```python
from build123d import *

# Parameters (mm, degrees)
SKETCH1_W           = 31.75
SKETCH1_H           = 8
SKETCH1_R           = 2.1
BOSS_EXTRUDE1_DEPTH = 21
SKETCH4_R           = 2.1
CUT_EXTRUDE3_DEPTH  = 38.5
SKETCH6_R           = 2.1
BOSS_EXTRUDE3_DEPTH = 2
SKETCH7_R           = 2.1
BOSS_EXTRUDE4_DEPTH = 2


with BuildPart() as part:
    # Sketch1 → Boss-Extrude1 (new body)
    with BuildSketch(Plane(origin=(0, 0, 0), x_dir=(1, 0, 0), z_dir=(0, 1, 0))):
        with Locations((4.725, 0)):
            Rectangle(SKETCH1_W, SKETCH1_H)
        with Locations(Location((0, 0, 0), (0, 0, 90))):
            Circle(SKETCH1_R, mode=Mode.SUBTRACT)
        with Locations(Location((-7.15, 0, 0), (0, 0, 90))):
            Circle(SKETCH1_R, mode=Mode.SUBTRACT)
        with Locations(Location((9.45, 0, 0), (0, 0, 90))):
            Circle(SKETCH1_R, mode=Mode.SUBTRACT)
        with Locations(Location((16.6, 0, 0), (0, 0, 90))):
            Circle(SKETCH1_R, mode=Mode.SUBTRACT)
    extrude(amount=BOSS_EXTRUDE1_DEPTH)

    # Sketch4 → Cut-Extrude3 (cut)
    with BuildSketch(Plane(origin=(20.6, 0, 0), x_dir=(0, 0, -1), z_dir=(1, 0, 0))):
        with Locations((0, 4)):
            Circle(SKETCH4_R)
    extrude(amount=-CUT_EXTRUDE3_DEPTH, mode=Mode.SUBTRACT)

    # Sketch6 → Boss-Extrude3 (add)
    with BuildSketch(Plane.XZ):
        with Locations(Location((-7.15, 0, 0), (0, 0, 90))):
            Circle(SKETCH6_R)
        with Locations(Location((0, 0, 0), (0, 0, 90))):
            Circle(SKETCH6_R)
        with Locations(Location((9.45, 0, 0), (0, 0, 90))):
            Circle(SKETCH6_R)
        with Locations(Location((16.6, 0, 0), (0, 0, 90))):
            Circle(SKETCH6_R)
    extrude(amount=-BOSS_EXTRUDE3_DEPTH)

    # Sketch7 → Boss-Extrude4 (add)
    with BuildSketch(Plane(origin=(20.6, 0, 0), x_dir=(0, 0, -1), z_dir=(1, 0, 0))):
        with Locations((0, 4)):
            Circle(SKETCH7_R)
    extrude(amount=-BOSS_EXTRUDE4_DEPTH)


solid = part.part
```
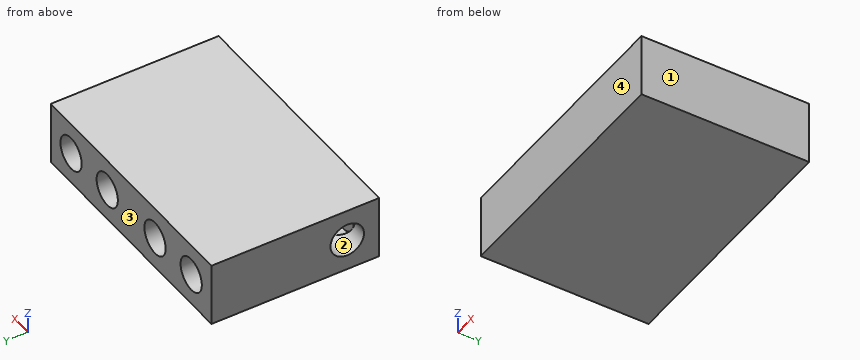
Input: part model. Units: mm. Frame: model coordinates. Face numbers are marked on the shaded views. Coordinates: 2 decimals unless noted, no trailing zeros. Write each loop counter-clockwise with the first axis right and the second up, starting at its lowest first coordinate (ties: lowest second). Pieces come first, ordered by that corner, then holes. Notation, with made-up numbers: (78, -2.75) -> (115, -2.75) arc R13 ccw to (115, 4.25) -> close; hole circle Ø4 at (-15.75, 78). An arc over 180 degrees is marked (long way). Answer as a JSON object with one key per item and string values.
1. Section A-A on y = 13.5. Return the cut outline in (x, z).
Result set:
{"outline": "(-11.15, -4) -> (20.6, -4) -> (20.6, 4) -> (-11.15, 4) -> close; hole circle Ø4.2 at (-7.15, 0); hole circle Ø4.2 at (0, 0); hole circle Ø4.2 at (9.45, 0); hole circle Ø4.2 at (16.6, 0)"}
2. Material intervals for line 1 (X direction, y = 11, z = 0); line 2 (Z direction, x = 15, y = 4); line 3 (X direction, y = 9.5, z = 0.5), sorted ascending. Write a range as from..to.
Result set:
{"line 1": "x = -11.15..-9.25, -5.05..-2.1, 2.1..7.35, 11.55..14.5, 18.7..20.6", "line 2": "z = -4..-2.1, 2.1..4", "line 3": "x = -11.15..-9.19, -5.11..-2.04, 2.04..7.41, 11.49..14.56, 18.64..20.6"}
3. Section D-D on z = 0. Count the separate pieces of the cut face and the enclosed holes in it, then the cut area to 3 significant figures.
Result set:
{"separate pieces": "5", "enclosed holes": "0", "area": "293 mm2"}
4. Section C-C on y = 3. Return the cut outline in (x, z).
Result set:
{"outline": "(-11.15, -4) -> (20.6, -4) -> (20.6, 4) -> (-11.15, 4) -> (-11.15, 1.85) -> (-8.15, 1.85) arc R2.1 cw to (-6.15, 1.85) -> (-1, 1.85) arc R2.1 cw to (1, 1.85) -> (8.45, 1.85) arc R2.1 cw to (10.45, 1.85) -> (15.6, 1.85) arc R2.1 cw to (17.6, 1.85) -> (18.6, 1.85) -> (18.6, -1.85) -> (17.6, -1.85) arc R2.1 cw to (15.6, -1.85) -> (10.45, -1.85) arc R2.1 cw to (8.45, -1.85) -> (1, -1.85) arc R2.1 cw to (-1, -1.85) -> (-6.15, -1.85) arc R2.1 cw to (-8.15, -1.85) -> (-11.15, -1.85) -> close"}
5. First-contact query: P1, Ø3.5, axis at x = 9.5, z = -0.5, coming from the +Y side; P2, Ø1.2, axis at y = 4, z = 1, coming from the -X side; P3, Ø3.5, axis at x = 16.6, z = 0, coming from the +Y side. Flat tips, straight axial feed; report the tip coordinate or a pass-through.
Result set:
{"P1": "stops at y = 21", "P2": "stops at x = 18.6", "P3": "stops at y = 2"}
6. Mould query, pull axis Y, two halves, no side actions, for the marked faces 1, 2, 3 and 4. Classes: released by +Y, released by -Y, zero draft, split by the parting line, or undercut.
Result set:
{"face 1": "zero draft", "face 2": "undercut", "face 3": "released by +Y", "face 4": "released by -Y"}
7. Section B-B on x = 14. Return the cut outline in (y, z).
Result set:
{"outline": "(0, -4) -> (21, -4) -> (21, 4) -> (0, 4) -> close; hole circle Ø4.2 at (4, 0)"}
